CAD build for the part. Positions are in the model's coordinates, mm. Face numbers are marked on the shaded views. Round coordinates to 2 decimals unless told otherwise and drop trailing zeros. Loops run counter-clockwise (first coordinate to the right, second up) from the corner with the lowest first, then second, coordinate; pieces in that order, holes last. Notation, with made-up numbers: M 81.5,-38 L 89.5,-38 A33 cw 89.5,-1 Z; hole C -3,69.25 d9. An arc over 180 degrees is marked long. Use one line per item in the form item = value.
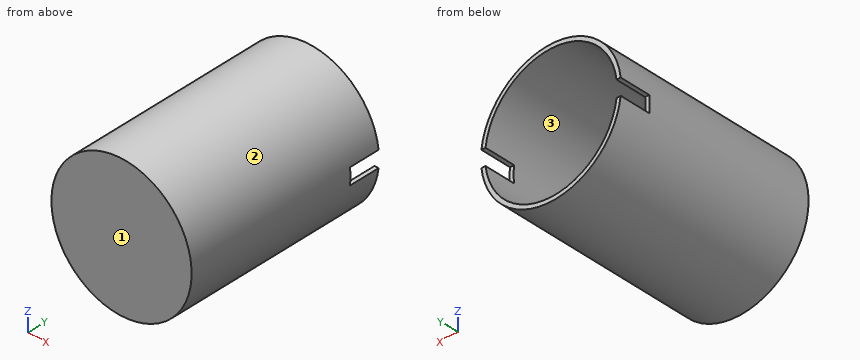
Autodesk Inventor part; units mm, degrees
ref_plane "YZ Plane" through (0, 0, 0) normal (1, 0, 0) x (0, 1, 0)
ref_plane "XZ Plane" through (0, 0, 0) normal (0, 1, 0) x (-1, 0, 0)
ref_plane "XY Plane" through (0, 0, 0) normal (0, 0, 1) x (1, 0, 0)
sketch "Sketch2" plane through (0, 0, 0) normal (0, 1, 0) x (-1, 0, 0)
  circle A0 centre (0, 0) radius 13.8
  line L0 (0, -13.8) -> (0, -13)
  dimension "d0" = 27.6
  dimension "d79" = 0.8
extrude "Extrusion1" add sketch "Sketch2" along normal blind 40
sketch "Sketch3" plane through (0, 40, 0) normal (0, 1, 0) x (1, 0, 0)
  circle A0 centre (0, 0) radius 13
  dimension "d3" = 26
hole "Hole1" at (0, 40, 0) direction (0, -1, 0) diameter 26 depth 39
sketch "Sketch8" plane through (0, 40, 0) normal (0, 1, 0) x (1, 0, 0)
  circle A0 centre (0, 0) radius 13.8
  line L0 (-13.8, 0) -> (-13.8, 1.6)
  line L1 (-13.8, 0) -> (-12.2, 0) construction
  line L2 (-13.8, 1.6) -> (-10.8, 1.6)
  line L3 (-10.8, 1.6) -> (-10.8, -1.6)
  line L4 (-10.8, -1.6) -> (-13.8, -1.6)
  line L5 (-13.8, -1.6) -> (-13.8, 0)
  point P0 (-13.7069, 1.6)
  point P1 (-13.7069, -1.6)
  dimension "d64" = 1.6
  dimension "d66" = 3
  dimension "d67" = 3.2
  dimension "d69" = 3
extrude "Extrusion6" cut sketch "Sketch8" against normal blind 6.1 contours L2 L3 L4 A0 picked at (-11.8, 0)
sketch "Sketch9" plane through (0, 40, 0) normal (0, 1, 0) x (1, 0, 0)
  circle A0 centre (0, 0) radius 13.8
  line L0 (13.8, 0) -> (13.8, 1.6)
  line L1 (13.8, 0) -> (15.4, 0) construction
  line L2 (13.8, 1.6) -> (10.8, 1.6)
  line L3 (10.8, 1.6) -> (10.8, -1.6)
  line L4 (10.8, -1.6) -> (13.8, -1.6)
  line L5 (13.8, -1.6) -> (13.8, 0)
  point P0 (13.7069, -1.6)
  point P1 (13.7069, 1.6)
  dimension "d72" = 1.6
  dimension "d74" = 3
  dimension "d75" = 3.2
  dimension "d76" = 3
extrude "Extrusion7" cut sketch "Sketch9" against normal blind 6.1 contours A0 L4 L3 L2 picked at (11.8, 0)
properties part number "Part6_containter_top" material "ABS Plastic"
1. Probe line 1 along X through (y, z) = (22.5, 0); line 2 along Z through (x, y) = (-0.5, 33.5); line 3 along Y through (x, z) = (-1.75, -2.25). List the from-to ranges inside material, lowest first. Write a range as from..to.
Completed:
line_1 = -13.8..-13, 13..13.8
line_2 = -13.79..-12.99, 12.99..13.79
line_3 = 0..1
2. Pull direction Z, two halves, no side cores. Call the marked faces 1, 2 and 3: +Z half, -Z half, draft (parallel to the pull), parting line (faces both ways), or undercut.
Completed:
face_1 = draft
face_2 = parting line
face_3 = undercut
3. Cut at B-B on y = 11.5. Write the cut outline in (x, z), and give its area (3 significant figures).
Completed:
outline = C 0,0 d27.6; hole C 0,0 d26
area = 67.4 mm2
4. Cut at C-C on x = 0. Write the cut outline in (y, z), and give its area (3 significant figures).
Completed:
outline = M 0,-13.8 L 40,-13.8 L 40,-13 L 1,-13 L 1,13 L 40,13 L 40,13.8 L 0,13.8 Z
area = 90.0 mm2
5. Cut at A-A on z = 0. Write the cut outline in (x, y).
Completed:
outline = M -13.8,0 L 13.8,0 L 13.8,33.9 L 13,33.9 L 13,1 L -13,1 L -13,33.9 L -13.8,33.9 Z
6. Drop flat-ended pins along their axis: P1, Ø1.5, axis at x = -2.5, z = -7.5, coming from the +Y side; P2, Ø1, axis at x = -13.5, z = 0.5, coming from the +Y side; P3, Ø6, axis at y = 25, z = 8, coming from the +X side. Give the stop position or say it passes through.
Completed:
P1 = 1
P2 = 33.9
P3 = 12.86
